For this review, take the finished solid that the model builds, in its own axes (mm). Round coordinates to 2 decimals unless told otherwise and drop trailing zeros. Write each loop counter-clockwise with the first axis right and the second up, starting at its lowest first coordinate (ties: lowest second). Pieces come first, ordered by that corner, then holes.
from build123d import *

# Parameters (mm, degrees)
SKETCH1_R           = 7
SKETCH1_R_2         = 2.5
BOSS_EXTRUDE1_DEPTH = 15


with BuildPart() as part:
    # Sketch1 → Boss-Extrude1 (new body)
    # profile 1 of 3: a face of its own
    with BuildSketch(Plane(origin=(0, 0, 0), x_dir=(1, 0, 0), z_dir=(0, 1, 0))):
        with BuildLine():
            Line((0, 7), (-131, 7))
            ThreePointArc((-131, 7), (-126.050252532, 4.949747468), (-124, 0))
            ThreePointArc((-124, 0), (-126.050252532, -4.949747468), (-131, -7))
            Line((-131, -7), (-55.118468675, -7))
            Line((-55.118468675, -7), (0, -7))
            ThreePointArc((0, -7), (-7, 0), (0, 7))
        make_face()
    # profile 2 of 3: a face of its own
    with BuildSketch(Plane(origin=(0, 0, 0), x_dir=(1, 0, 0), z_dir=(0, 1, 0))):
        with Locations((-131, 0)):
            Circle(SKETCH1_R)
        with Locations(Location((-131, 0, 0), (0, 0, 270))):
            Circle(SKETCH1_R_2, mode=Mode.SUBTRACT)
    # profile 3 of 3: a face of its own
    with BuildSketch(Plane(origin=(0, 0, 0), x_dir=(1, 0, 0), z_dir=(0, 1, 0))):
        Circle(SKETCH1_R)
        with Locations(Location((0, 0, 0), (0, 0, 270))):
            Circle(SKETCH1_R_2, mode=Mode.SUBTRACT)
    extrude(amount=BOSS_EXTRUDE1_DEPTH)


solid = part.part
(1) For line 1 along X through (y, z) = (11.75, 0); line 2 along Z through (x, y) = (-131, 4); line 3 along X through (y, z) = (1.5, -1.25), list the stretches that pass through material, from the lowest coordinate up.
Geometry check:
line 1: x = -138 to -133.5, -128.5 to -2.5, 2.5 to 7
line 2: z = -7 to -2.5, 2.5 to 7
line 3: x = -137.89 to -133.17, -128.83 to -2.17, 2.17 to 6.89
(2) We need section B-B, the plane y = 3.5. Give the boundary of the cut face in (x, z).
Geometry check:
outline: (-131, -7) - (0, -7) arc R7 ccw to (0, 7) - (-131, 7) arc R7 ccw to start; hole circle Ø5 at (-131, 0); hole circle Ø5 at (0, 0)
(3) We need section C-C, the plane z = -5.75. Give the boundary of the cut face in (x, y).
Geometry check:
outline: (-134.99, 0) - (3.99, 0) - (3.99, 15) - (-134.99, 15) - close
(4) We need section A-A, the plane z = 0. Give the boundary of the cut face in (x, y).
Geometry check:
outline: (-138, 0) - (-133.5, 0) - (-133.5, 15) - (-138, 15) - close; (-128.5, 0) - (-2.5, 0) - (-2.5, 15) - (-128.5, 15) - close; (2.5, 0) - (7, 0) - (7, 15) - (2.5, 15) - close
(5) Mouldability with a two-part tool opening along Z and no side actions: class faces 1 (the face through (-66, 7, 7)), 2 (the face through (-67, 0, 0)), 3 (the face through (-128.52, 7.4, -0.33)) as pulls with the +Z half, pulls with the -Z half, needs draft (parallel to the pull), parting line crosses it, or undercut.
Geometry check:
face 1: pulls with the +Z half
face 2: needs draft
face 3: undercut
(6) For pin 1 Ø8 at (y, z) = (1.5, -3) entering from -X, flat-tipped, find the tip position at first contact; note if it passes through.
Geometry check:
pin 1: stops at x = -138
